from build123d import *

# Parameters (mm, degrees)
SKETCH1_W           = 127
SKETCH1_H           = 76.2
BOSS_EXTRUDE1_DEPTH = 6.35
SKETCH3_R           = 14.2875
CUT_EXTRUDE1_DEPTH  = 75.324844433
SKETCH4_R           = 11.1125
CUT_EXTRUDE2_DEPTH  = 75.324844433


with BuildPart() as part:
    # Sketch1 → Boss-Extrude1 (new body)
    with BuildSketch(Plane(origin=(0, 0, 0), x_dir=(1, 0, 0), z_dir=(0, 1, 0))):
        Rectangle(SKETCH1_W, SKETCH1_H)
    extrude(amount=BOSS_EXTRUDE1_DEPTH)

    # Sketch3 → Cut-Extrude1 (cut, through all)
    with BuildSketch(Plane(origin=(0, 6.35, 0), x_dir=(1, 0, 0), z_dir=(0, 1, 0))):
        with Locations(Location((-15.875, 0, 0), (0, 0, 270))):
            Circle(SKETCH3_R)
    extrude(amount=-CUT_EXTRUDE1_DEPTH, mode=Mode.SUBTRACT)

    # Sketch4 → Cut-Extrude2 (cut, through all)
    with BuildSketch(Plane(origin=(0, 6.35, 0), x_dir=(1, 0, 0), z_dir=(0, 1, 0))):
        with Locations(Location((15.875, 0, 0), (0, 0, 270))):
            Circle(SKETCH4_R)
    extrude(amount=-CUT_EXTRUDE2_DEPTH, mode=Mode.SUBTRACT)


solid = part.part
The listing builds one solid part. Answer for the finished solid, in the listing's coordinates (mm). Give positions to 0.01 mm unless a question says otherwise; leave off trailing zeros. Order: outer loops, then holes, each group sorted by start corner. A loop starts at its lowest first (then second) coordinate and runs counter-clockwise, first axis right, second up. Notation, with made-up numbers: (3, -20) -> (20, -20) arc R18 cw to (20, 15) -> close; hole circle Ø6 at (8.5, 44). An arc over 180 degrees is marked (long way). Put each result on its own line as item: value.
Item 1: For a pull along X with two mould halves and no side action, classify faces 1 (the face through (-63.5, 3, 1)), 2 (the face through (-1, 3, -38.1)), 3 (the face through (26.9, 3.2, -1.4)) as released by +X, released by -X, zero draft, split by the parting line, or undercut.
Established:
face 1: released by -X
face 2: zero draft
face 3: undercut
Item 2: A cutting plane is placed at C-C on y = 2.5. Give the vertices of the cut face in (x, z) (1 decimal), plus the area to 3 significant figures.
Established:
outline: (-63.5, -38.1) -> (63.5, -38.1) -> (63.5, 38.1) -> (-63.5, 38.1) -> close; hole circle Ø28.6 at (-15.9, 0); hole circle Ø22.2 at (15.9, 0)
area: 8,650 mm^2
Item 3: A cutting plane is placed at B-B on x = -23. Give the vertices of the cut face in (y, z).
Established:
outline: (0, -38.1) -> (6.35, -38.1) -> (6.35, -12.38) -> (0, -12.38) -> close; (0, 12.38) -> (6.35, 12.38) -> (6.35, 38.1) -> (0, 38.1) -> close
Item 4: A cutting plane is placed at D-D on x = -8. Give the vertices of the cut face in (y, z), plus the area to 3 significant figures.
Established:
outline: (0, -38.1) -> (6.35, -38.1) -> (6.35, -11.92) -> (0, -11.92) -> close; (0, 11.92) -> (6.35, 11.92) -> (6.35, 38.1) -> (0, 38.1) -> close
area: 332 mm^2
Item 5: Straight lines are drawn through the part: line 1 (X direction, y = 4.75, z = 0); line 2 (Z direction, x = -15, y = 5); line 3 (X direction, y = 2.25, z = -2). For each, find the intervals that lie inside material, in ascending order.
Established:
line 1: x = -63.5 to -30.16, -1.59 to 4.76, 26.99 to 63.5
line 2: z = -38.1 to -14.26, 14.26 to 38.1
line 3: x = -63.5 to -30.02, -1.73 to 4.94, 26.81 to 63.5
Item 6: A cutting plane is placed at A-A on z = 0. Give the vertices of the cut face in (x, y).
Established:
outline: (-63.5, 0) -> (-30.16, 0) -> (-30.16, 6.35) -> (-63.5, 6.35) -> close; (-1.59, 0) -> (4.76, 0) -> (4.76, 6.35) -> (-1.59, 6.35) -> close; (26.99, 0) -> (63.5, 0) -> (63.5, 6.35) -> (26.99, 6.35) -> close
